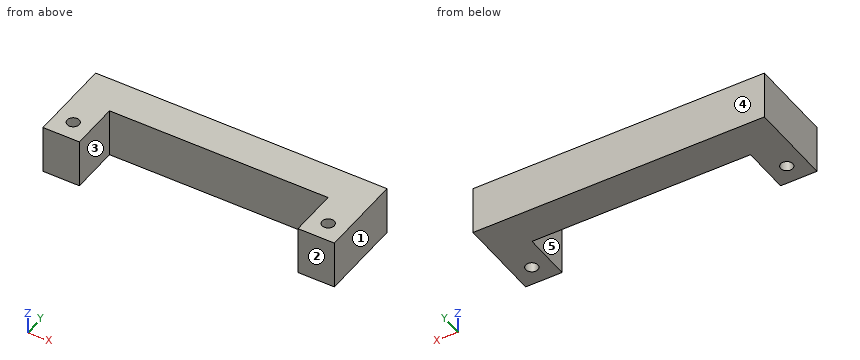
Autodesk Inventor part; units mm, degrees
ref_plane "YZ Plane" through (0, 0, 0) normal (1, 0, 0) x (0, 1, 0)
ref_plane "XZ Plane" through (0, 0, 0) normal (0, 1, 0) x (-1, 0, 0)
ref_plane "XY Plane" through (0, 0, 0) normal (0, 0, 1) x (1, 0, 0)
sketch "Sketch1" plane through (0, 0, 0) normal (0, 0, 1) x (1, 0, 0)
  line L0 (-60, 7.5) -> (60, 7.5)
  line L1 (60, 7.5) -> (60, -7.5)
  line L2 (60, -7.5) -> (-60, -7.5)
  line L3 (-60, -7.5) -> (-60, 7.5)
  line L4 (-60, 7.5) -> (60, -7.5) construction
  line L5 (60, 7.5) -> (-60, -7.5) construction
  line L6 (-60, -7.5) -> (-45, -7.5)
  line L7 (-45, -7.5) -> (-45, -27.5)
  line L8 (-45, -27.5) -> (-60, -27.5)
  line L9 (-60, -27.5) -> (-60, -7.5)
  line L10 (60, -7.5) -> (45, -7.5)
  line L11 (45, -7.5) -> (45, -27.5)
  line L12 (45, -27.5) -> (60, -27.5)
  line L13 (60, -27.5) -> (60, -7.5)
  circle A0 centre (-52.5, -19.5) radius 2.5
  circle A1 centre (52.5, -19.5) radius 2.5
  point P0 (0, 0)
  dimension "d17" = 120
  dimension "d18" = 15
  dimension "d19" = 15
  dimension "d20" = 20
  dimension "d21" = 15
  dimension "d22" = 20
  dimension "d23" = 5
  dimension "d24" = 5
extrude "Extrusion1" add sketch "Sketch1" along normal blind 20
properties part number "front_U_shaped_frame[1]"
Build history of the part. All positions in model axes, mm. Face numbers are marked on the shaded views. A direction names the side the tool comes from. Round coordinates to 2 decimals unless told otherwise and drop trailing zeros. Write each loop counter-clockwise with the first axis right and the second up, starting at its lowest first coordinate (ties: lowest second). Pieces come first, ordered by that corner, then holes. Notation, with made-up numbers: M 65.5,-26 L 78.5,-26 A37 ccw 78.5,13 Z; hole C 24.25,-4.75 d7. An arc over 180 degrees is marked long. Use CSV: the item, a comma, the result in double quotes.
1. Wall check: probe 1 along Y at (x, z) = (-52.5, 9.75); probe 2 along X at (y, z) = (-18, 14.25); probe 3 along X at (y, z) = (-12, 16.5). Give the ranges that are in metal, low to high. Write a range as from..to.
Reply:
probe 1,"y = -27.5..-22, -17..7.5"
probe 2,"x = -60..-54.5, -50.5..-45, 45..50.5, 54.5..60"
probe 3,"x = -60..-45, 45..60"
2. Saw through at A-A (y = -19.5). Give the cut face in (x, z).
Reply:
outline,"M -60,0 L -55,0 L -55,20 L -60,20 Z; M -50,0 L -45,0 L -45,20 L -50,20 Z; M 45,0 L 50,0 L 50,20 L 45,20 Z; M 55,0 L 60,0 L 60,20 L 55,20 Z"
3. Tool access for the marked faces 4 and 5: list every direction of +Z, -Z, +X, -X, +Y, -Y with a clear straight run to the whole face (end or side of a thin tool).
Reply:
face 4,"+Z, -Z, +X, -X, +Y"
face 5,"+Z, -Z, -Y"
4. Saw through at C-C (x = 52.5). Give the cut face in (y, z).
Reply:
outline,"M -27.5,0 L -22,0 L -22,20 L -27.5,20 Z; M -17,0 L 7.5,0 L 7.5,20 L -17,20 Z"
5. Saw through at B-B (y = -10). Give the cut face in (x, z).
Reply:
outline,"M -60,0 L -45,0 L -45,20 L -60,20 Z; M 45,0 L 60,0 L 60,20 L 45,20 Z"
6. Two-plate mould, pull along X, no slides. Class the marked faces 1, 2 and 3: +X half, -X half, draft (parallel to the pull), parting line (faces both ways), or undercut.
Reply:
face 1,"+X half"
face 2,"draft"
face 3,"undercut"
7. Flat gauge pin, fed straight in: pin 1 (8 mm diameter, centred on x = 24.5, z = 7.5, fed in from -Y). Where does the tip first touch, or does it go through?
Reply:
pin 1,"stops at y = -7.5"
8. Saw through at D-D (z = 18.25). Give the cut face in (x, y), plus the area to 3 significant figures.
Reply:
outline,"M -60,-27.5 L -45,-27.5 L -45,-7.5 L 45,-7.5 L 45,-27.5 L 60,-27.5 L 60,7.5 L -60,7.5 Z; hole C -52.5,-19.5 d5; hole C 52.5,-19.5 d5"
area,"2,360 mm²"
